Verification items for the finished model (mm, model axes). A direction names the side the tool comes from. Round coordinates to 2 decimals unless told otherwise and drop trailing zeros. Write each loop counter-clockwise with the first axis right and the second up, starting at its lowest first coordinate (ties: lowest second). Pieces come first, ordered by that corner, then holes.
from build123d import *

# Parameters (mm, degrees)
F0_R     = 4.75
F1_DEPTH = 15
F2_R     = 1.5
F3_DEPTH = 7.5
F4_R     = 2
F5_DEPTH = 7.5
F8_D     = 3.5
F8_DEPTH = 5
F8_TIP   = 1.0515060833
F9_D     = 3.5
F9_DEPTH = 5
F9_TIP   = 1.0515060833


with BuildPart() as f1:
    # F0 (on Top) → F1 (new body)
    with BuildSketch(Plane.XY):
        Circle(F0_R)
    extrude(amount=F1_DEPTH)

    # F2 (on face) → F3 (cut)
    with BuildSketch(Plane.XY.offset(15)):
        Circle(F2_R)
    extrude(amount=-F3_DEPTH, mode=Mode.SUBTRACT)

    # F4 (on Top) → F5 (cut)
    with BuildSketch(Plane.XY):
        Circle(F4_R)
    extrude(amount=F5_DEPTH, mode=Mode.SUBTRACT)

    # F8 (one way)
    with BuildSketch(Plane.XZ):
        with Locations((0, 11)):
            Circle(F8_D / 2)
    extrude(amount=-F8_DEPTH, mode=Mode.SUBTRACT)
    with Locations(Plane.XZ):
        with Locations((0, 11)):
            with Locations((0, 0, -(F8_DEPTH + F8_TIP / 2))):  # 118° drill point
                Cone(0, F8_D / 2, F8_TIP, mode=Mode.SUBTRACT)

    # F9 (one way)
    with BuildSketch(Plane.XZ):
        with Locations((0, 4)):
            Circle(F9_D / 2)
    extrude(amount=-F9_DEPTH, mode=Mode.SUBTRACT)
    with Locations(Plane.XZ):
        with Locations((0, 4)):
            with Locations((0, 0, -(F9_DEPTH + F9_TIP / 2))):  # 118° drill point
                Cone(0, F9_D / 2, F9_TIP, mode=Mode.SUBTRACT)


solid = f1.part
Q1. Sectioned sample at B-B (z = 6.25). Enter the section's corners in (x, y), plus the area to 3 significant figures.
Recorded:
outline: circle Ø9.5 at (0, 0); hole circle Ø4 at (0, 0)
area: 58.3 mm2
Q2. Tool access check on faces 1 (the cylindrical face through (1.617, 2.871, 10.33)), 2 (the cylindrical face through (-0.325, -1.464, 11.302)). Record the directions out of +Z, -Z, +X, -X, +Y, -Y that give a thin tool (end or side, any length) a straight path to the whole face; none if there is none.
Recorded:
face 1: +Y
face 2: +Z, -Z
Q3. Sectioned sample at C-C (y = 3.5). Enter the section's corners in (x, z), plus the area to 3 significant figures.
Recorded:
outline: (-3.21, 0) - (3.21, 0) - (3.21, 15) - (-3.21, 15) - close; hole circle Ø3.5 at (0, 4); hole circle Ø3.5 at (0, 11)
area: 77.1 mm2
Q4. Depth check by flat-ended pin: P1, Ø1, axis at y = 1, z = 6.5, coming from the +X side. Enter the tip coordinate at first touch or a pass-through.
Recorded:
P1: stops at x = 4.72
Q5. Sectioned sample at A-A (x = 0). Enter the section's corners in (y, z), plus the area to 3 significant figures.
Recorded:
outline: (-4.75, 0) - (-2, 0) - (-2, 7.5) - (-1.5, 7.5) - (-1.5, 15) - (-4.75, 15) - close; (1.5, 7.5) - (2, 7.5) - (2, 5.75) - (4.75, 5.75) - (4.75, 9.25) - (1.5, 9.25) - close; (1.5, 12.75) - (4.75, 12.75) - (4.75, 15) - (1.5, 15) - close; (2, 0) - (4.75, 0) - (4.75, 2.25) - (2, 2.25) - close
area: 69.0 mm2
Q6. Sectioned sample at D-D (x = 1). Enter the section's corners in (y, z).
Recorded:
outline: (-4.64, 0) - (-1.73, 0) - (-1.73, 7.5) - (-1.12, 7.5) - (-1.12, 15) - (-4.64, 15) - close; (1.12, 7.5) - (1.73, 7.5) - (1.73, 5.44) - (4.64, 5.44) - (4.64, 9.56) - (1.12, 9.56) - close; (1.12, 12.44) - (4.64, 12.44) - (4.64, 15) - (1.12, 15) - close; (1.73, 0) - (4.64, 0) - (4.64, 2.56) - (1.73, 2.56) - close
Q7. Release check for a two-part mould opening along X. For faces 3 (the cylindrical face through (-1.03, -4.637, 7.395)), 4 (the cylindrical face through (0, -2, 4)), 5 (the flat face through (2, 0, 15)) record: released by +X, released by -X, zero draft, split by the parting line, or undercut.
Recorded:
face 3: split by the parting line
face 4: undercut
face 5: zero draft
Q8. Material ranges on line 1 along Z through (x, y) = (0, 3.9); line 2 along Z through (x, y) = (-0.75, 3.5); line 3 along X through (y, z) = (1.75, 1.5), recorded low to high.
Recorded:
line 1: z = 0 to 2.25, 5.75 to 9.25, 12.75 to 15
line 2: z = 0 to 2.42, 5.58 to 9.42, 12.58 to 15
line 3: x = -4.42 to -0.97, 0.97 to 4.42
